Could you check a few things on this model? Use its own coordinates, in mm. Face numbers are marked on the shaded views. A direction names the side the tool comes from. Give positions to 0.01 mm unless a question says otherwise; leave off trailing zeros. Loops run counter-clockwise (first coordinate to the right, second up) from the corner with the lowest first, then second, coordinate; pieces in that order, holes last. Notation, with made-up numbers: (26, -4) -> (70, -4) arc R23 ccw to (70, 23) -> close; hole circle Ø4 at (88, 20.5). An arc over 180 degrees is marked (long way). Put each result on its own line as item: value.
Autodesk Inventor part; units mm, degrees
ref_plane "YZ Plane" through (0, 0, 0) normal (1, 0, 0) x (0, 1, 0)
ref_plane "XZ Plane" through (0, 0, 0) normal (0, 1, 0) x (-1, 0, 0)
ref_plane "XY Plane" through (0, 0, 0) normal (0, 0, 1) x (1, 0, 0)
sketch "Sketch1" plane through (0, 0, 0) normal (0, 0, 1) x (1, 0, 0)
  line L0 (0, 0) -> (0, 40.244)
  line L1 (-5.08, 41.6052) -> (-5.08, 0)
  line L2 (-5.08, 0) -> (0, 0)
  line L3 (-5.08, 41.6052) -> (14.2875, 75.1507)
  line L4 (14.2875, 75.1507) -> (-9.646, 116.6048)
  line L5 (-9.646, 116.6048) -> (-5.2466, 119.1448)
  line L6 (-5.2466, 119.1448) -> (20.1534, 75.1507)
  line L7 (20.1534, 75.1507) -> (0, 40.244)
  line L8 (-5.2466, 119.1448) -> (-0.1666, 100.186)
  dimension "d0" = 41.6052
  dimension "d1" = 5.08
  dimension "d6" = 5.08
  dimension "d7" = 5.08
  dimension "d8" = 30
  dimension "d10" = 120
  dimension "d11" = 50.8
  dimension "d12" = 38.735
  dimension "d13" = 15
extrude "Extrusion1" add sketch "Sketch1" along normal blind 20.32 contours L2 L1 L3 L4 L8 L6 L7 L0
fillet "Fillet1" radius 1.5875 1 edges at (-5.2466, 119.1448, 10.16)
ref_plane "Work Plane1" through (-10.16, 0, 0) normal (-1, 0, 0) x (0, 0, 1)
sketch "Sketch2" plane through (-10.16, 0, 0) normal (-1, 0, 0) x (0, 0, 1)
  line L0 (0, 0) -> (20.32, 0)
  line L1 (3.937, 0) -> (16.383, 0)
  line L2 (16.383, 0) -> (16.383, 50.3936)
  line L3 (16.383, 50.3936) -> (3.937, 50.3936)
  line L4 (3.937, 50.3936) -> (3.937, 0)
  point P0 (10.16, 0)
  dimension "d16" = 12.446
  dimension "d17" = 50.3936
  dimension "d18" = 6.223
extrude "Extrusion2" add sketch "Sketch2" against normal up to next
sketch "Sketch3" plane through (0, 0, 0) normal (1, 0, 0) x (0, 0, -1)
  circle A0 centre (-10.16, 20.122) radius 1.778
  line L0 (0, 0) -> (0, 40.244)
  line L1 (0, 0) -> (-20.32, 0)
  point P0 (0, 20.122)
  point P1 (-10.16, 0)
  dimension "d21" = 3.556
extrude "Extrusion3" cut sketch "Sketch3" against normal blind 25.4
sketch "Sketch4" plane through (0, 0, 0) normal (1, 0, 0) x (0, 0, -1)
  circle A0 centre (-10.16, 20.122) radius 1.778
  circle A1 centre (-10.16, 20.122) radius 3.81
  point P0 (0, 0)
  dimension "d24" = 7.62
extrude "Extrusion4" cut sketch "Sketch4" against normal blind 4.0132
properties part number "KNUCKLE 2"
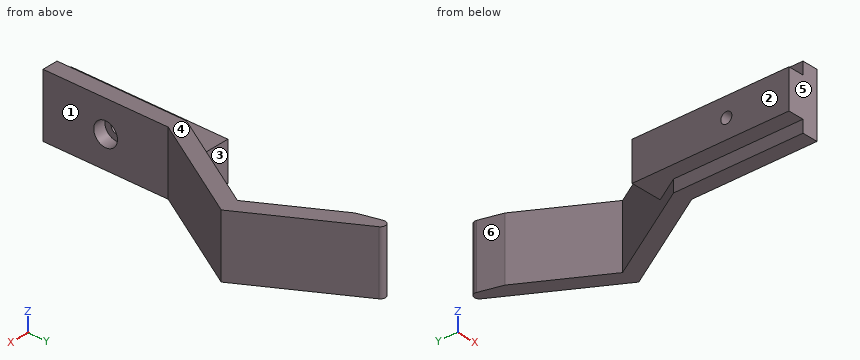
1. I need wall thicknesses on line 1 (Y direction, x = -7, z = 10.16); line 2 (Y direction, x = -3.2, z = 10.16); line 3 (X direction, y = 15, z = 5.5). Which ranges of each line are inside material? Lowest first, please.
Recorded:
line 1: y = 0 to 18.34, 21.9 to 50.39
line 2: y = 0 to 16.31, 23.93 to 50.39
line 3: x = -10.16 to 0
2. I'm going to push flat-ended pins straight in: pin 1 (4 mm diameter, centred on y = 20.122, z = 10.16, fed in from +X); pin 2 (4 mm diameter, centred on x = 17, z = 7.5, fed in from -Y); pin 3 (4 mm diameter, centred on x = 11.5, z = 4.5, fed in from -Y). Where does each tip first touch, or does it pass through?
Recorded:
pin 1: stops at x = -4.01
pin 2: stops at y = 66.22
pin 3: stops at y = 56.7
3. If we section it at D-D (y = 60): List the corners of the cut face in (x, z) for me.
Recorded:
outline: (5.54, 0) -> (11.41, 0) -> (11.41, 20.32) -> (5.54, 20.32) -> close
4. If we section it at B-B (x = 8): List the corners of the cut face in (y, z) for me.
Recorded:
outline: (54.1, 0) -> (64.26, 0) -> (64.26, 20.32) -> (54.1, 20.32) -> close; (86.04, 0) -> (96.2, 0) -> (96.2, 20.32) -> (86.04, 20.32) -> close
5. If we section it at A-A (z = 10.16): List the corners of the cut face in (x, y) for me (1 decimal), then the cut area to 3 significant figures.
Recorded:
outline: (-10.2, 0) -> (0, 0) -> (0, 16.3) -> (-4, 16.3) -> (-4, 18.3) -> (-10.2, 18.3) -> close; (-10.2, 21.9) -> (-4, 21.9) -> (-4, 23.9) -> (0, 23.9) -> (0, 40.2) -> (20.2, 75.2) -> (0.8, 108.7) arc R1.6 ccw to (-2.1, 107.5) -> (-0.2, 100.2) -> (14.3, 75.2) -> (0, 50.4) -> (-10.2, 50.4) -> close
area: 821 mm^2
6. Thinking about a two-plate mould opening in Y: for the marked faces 4, 5 and 6, which applies, pulls with the +Y half, pulls with the -Y half, needs draft (parallel to the pull), parting line crosses it, or undercut?
Recorded:
face 4: needs draft
face 5: pulls with the -Y half
face 6: undercut
7. If we section it at C-C (x = -6.5): List the corners of the cut face in (y, z) for me.
Recorded:
outline: (0, 3.94) -> (50.39, 3.94) -> (50.39, 16.38) -> (0, 16.38) -> close; hole circle Ø3.56 at (20.12, 10.16)
8. For the marked faces 1, 2 and 3, which set-ups out of +Z, -Z, +X, -X, +Y, -Y let a thin tool reach every point of the face, with its end or its side?
Recorded:
face 1: +Z, -Z, +X, -Y
face 2: +Z, -Z, -X, +Y, -Y
face 3: +Z, -Z, -X
